Verification items for the finished model (mm, model axes). Coordinates: 2 decimals unless noted, no trailing zeros. Order: outer loops, then holes, each group sorted by start corner. A loop starts at its lowest first (then second) coordinate and runs counter-clockwise, first axis right, second up. Notation, with made-up numbers: (6, 23) -> (41, 23) arc R10 ccw to (41, 42) -> close; hole circle Ø10 at (-10, 86). An arc over 180 degrees is marked (long way). Write item = value, one per line. Start each with the question number.
1. Cross-section at B-B on y = 7.5. Record the cut outline in (x, z).
2. Cross-section at D-D on y = -68. Record the cut outline in (x, z), plus the area to 3 significant figures.
3. Thickness scan on line 1 along Y through (x, z) = (76.85, 0); line 2 along X through (y, z) = (-16.5, -3.5); line 3 along Z through (x, y) = (-78.5, 7.5). Record the ranges inside material, lowest first. Write a range as from..to.
4. Cross-section at C-C on y = -55. Record the cut outline in (x, z).
5. Cross-section at A-A on z = -6. Record the cut outline in (x, y) (3 decimals).
6. Go/stop test with flat-tipped pins: P1, Ø2, axis at x = -20.5, z = -0.5, coming from the +Y side; P2, Ø3, axis at y = -64.5, z = 3.5, coming from the -X side; P3, Ø4, axis at x = 74, z = -0.5, coming from the +Y side; P4, Ø4.5, axis at y = -7.5, z = 0, coming from the +X side. Record where each tip stops, or that it passes through.
from build123d import *

# Parameters (mm, degrees)
BOSS_EXTRUDE1_DEPTH                 = 4
BOSS_EXTRUDE2_DEPTH                 = 7.5
F_8_0_199_DIAMETER_HOLE1_AT_2_COUNT = 2
F_8_0_199_DIAMETER_HOLE1_AT_2_PITCH = 15


with BuildPart() as part:
    # Sketch1 → Boss-Extrude1 (new body, symmetric)
    with BuildSketch(Plane.XY):
        with BuildLine():
            Line((-68.014741233, -17.6), (-72.139067259, -17.6))
            ThreePointArc((-72.139067259, -17.6), (-71.75538681, -19.104174642), (-71.340346404, -20.6))
            ThreePointArc((-71.340346404, -20.6), (0, -74.255), (71.340346404, -20.6))
            ThreePointArc((71.340346404, -20.6), (71.75538681, -19.104174642), (72.139067259, -17.6))
            Line((72.139067259, -17.6), (68.014741233, -17.6))
            ThreePointArc((68.014741233, -17.6), (0, -70.255), (-68.014741233, -17.6))
        make_face()
    extrude(amount=BOSS_EXTRUDE1_DEPTH, both=True)

    # Sketch1_5 → Boss-Extrude2 (add, symmetric)
    with BuildSketch(Plane.XY):
        with BuildLine():
            ThreePointArc((-72.139067259, -17.6), (-71.75538681, -19.104174642), (-71.340346404, -20.6))
            Line((-71.340346404, -20.6), (-79.1, -20.6))
            Line((-79.1, -20.6), (-79.1, 17.5))
            Line((-79.1, 17.5), (-76.1, 17.5))
            Line((-76.1, 17.5), (-76.1, -17.6))
            Line((-76.1, -17.6), (-72.139067259, -17.6))
        make_face()
        with BuildLine():
            ThreePointArc((71.340346404, -20.6), (71.75538681, -19.104174642), (72.139067259, -17.6))
            Line((72.139067259, -17.6), (76.1, -17.6))
            Line((76.1, -17.6), (76.1, 17.5))
            Line((76.1, 17.5), (79.1, 17.5))
            Line((79.1, 17.5), (79.1, -20.6))
            Line((79.1, -20.6), (71.340346404, -20.6))
        make_face()
    extrude(amount=BOSS_EXTRUDE2_DEPTH, both=True)

    # Sketch4 → 8 _0.199_ Diameter Hole1 (revolve, cut)
    with BuildSketch(Plane(origin=(-79.1, 7.5, 0), x_dir=(0, 0, 1), z_dir=(0, 1, 0))):
        Polygon((0, 0), (0, 13), (2.5273, 11.481444958), (2.5273, 0), align=None)
    f_8_0_199_diameter_hole1 = revolve(axis=Axis((-85.45, 7.5, 0), (1, 0, 0)), mode=Mode.SUBTRACT)

    # 8 _0.199_ Diameter Hole1 at 2: 8 _0.199_ Diameter Hole1 ×2
    with Locations(*[(0, -i * F_8_0_199_DIAMETER_HOLE1_AT_2_PITCH, 0) for i in range(1, F_8_0_199_DIAMETER_HOLE1_AT_2_COUNT)]):
        add(f_8_0_199_diameter_hole1, mode=Mode.SUBTRACT)

    # Mirror1: 8 _0.199_ Diameter Hole1 across plane
    add(f_8_0_199_diameter_hole1.mirror(Plane(origin=(0, 0, 0), x_dir=(0, 0, 1), z_dir=(1, 0, 0))), mode=Mode.SUBTRACT)

    # Mirror1 copy 1 sketch → Mirror1 copy 1 (revolve, cut)
    with BuildSketch(Plane(origin=(79.1, -7.5, 0), x_dir=(0, 0, 1), z_dir=(0, 1, 0))):
        Polygon((0, 0), (0, -13), (2.5273, -11.481444958), (2.5273, 0), align=None)
    revolve(axis=Axis((85.45, -7.5, 0), (1, 0, 0)), mode=Mode.SUBTRACT)


solid = part.part
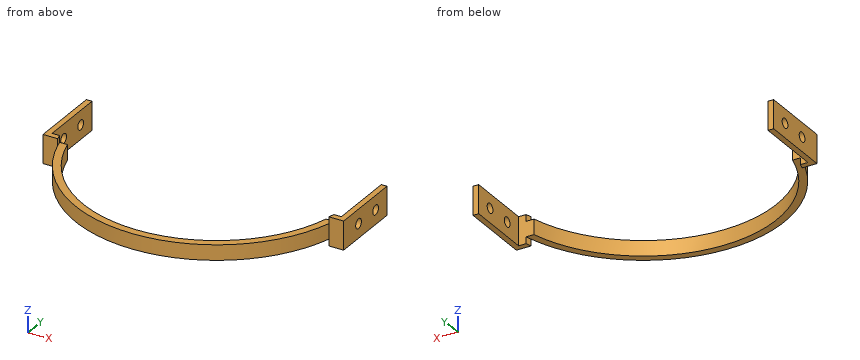
Worked out:
q1.outline = (-79.1, -7.5) -> (-76.1, -7.5) -> (-76.1, -2.53) -> (-79.1, -2.53) -> close; (-79.1, 2.53) -> (-76.1, 2.53) -> (-76.1, 7.5) -> (-79.1, 7.5) -> close; (76.1, -7.5) -> (79.1, -7.5) -> (79.1, -2.53) -> (76.1, -2.53) -> close; (76.1, 2.53) -> (79.1, 2.53) -> (79.1, 7.5) -> (76.1, 7.5) -> close
q2.outline = (-29.83, -4) -> (-17.66, -4) -> (-17.66, 4) -> (-29.83, 4) -> close; (17.66, -4) -> (29.83, -4) -> (29.83, 4) -> (17.66, 4) -> close
q2.area = 195 mm²
q3.line_1 = -20.6..-10.03, -4.97..4.97, 10.03..17.5
q3.line_2 = -79.1..-76.1, 76.1..79.1
q3.line_3 = -7.5..-2.53, 2.53..7.5
q4.outline = (-49.89, -4) -> (-43.71, -4) -> (-43.71, 4) -> (-49.89, 4) -> close; (43.71, -4) -> (49.89, -4) -> (49.89, 4) -> (43.71, 4) -> close
q5.outline = (-79.1, -20.6) -> (-71.34, -20.6) arc R74.255 cw to (-72.139, -17.6) -> (-76.1, -17.6) -> (-76.1, 17.5) -> (-79.1, 17.5) -> close; (71.34, -20.6) -> (79.1, -20.6) -> (79.1, 17.5) -> (76.1, 17.5) -> (76.1, -17.6) -> (72.139, -17.6) arc R74.255 cw to start
q6.P1 = -66.88
q6.P2 = -39.3
q6.P3 = -17.6
q6.P4 = through
